```python
from build123d import *

# Parameters (mm, degrees)
SKETCH_1_W      = 119.86
SKETCH_1_H      = 5.07
SKETCH_1_W_2    = 40.6
SKETCH_1_W_3    = 66.26
EXTRUDE_1_DEPTH = 5


with BuildPart() as part:
    # ｽｹｯﾁ1 → ﾎﾞｽ - 押し出し1 (new body)
    with BuildSketch(Plane.XY):
        Polygon((0, 25), (0, 0), (20, 0), (60.6, 0), (60.6, 5.93), (73.6, 5.93), (73.6, 0), (139.86, 0), (164.93, 0), (164.93, 25), (139.86, 25), (20, 25), align=None)
        with Locations((79.93, 27.535)):
            Rectangle(SKETCH_1_W, SKETCH_1_H)
        with Locations((40.3, -2.535)):
            Rectangle(SKETCH_1_W_2, SKETCH_1_H)
        with Locations((106.73, -2.535)):
            Rectangle(SKETCH_1_W_3, SKETCH_1_H)
    extrude(amount=EXTRUDE_1_DEPTH)


solid = part.part
```
Work out the finished part from the listing and answer in its coordinate system (mm). A direction names the side the tool comes from. Give positions to 0.01 mm unless a question says otherwise; leave off trailing zeros. Loops run counter-clockwise (first coordinate to the right, second up) from the corner with the lowest first, then second, coordinate; pieces in that order, holes last. Notation, with made-up numbers: (7, -15) -> (30, -15) arc R24 cw to (30, 13) -> close; hole circle Ø10 at (-5.75, 5). An arc over 180 degrees is marked (long way). Put each result on its own line as item: value. Start each with the question number.
Item 1: Find the intervals of material crossed by L1, parallel to X at y = 3, z = 0.75; L2, parallel to X at y = -3, z = 3.8; L3, parallel to X at y = 25.5, z = 3.75, in increasing order. Write a range as [from, to].
Item 2: The part is cut by section B-B (x = 154). Give the vertices of the cut face in (y, z).
Item 3: Each of these flat-tipped pins is pushed along its axis until it touches: P1, Ø1.5, axis at y = 28, z = 3.5, coming from the +X side; P2, Ø2.5, axis at y = 28.5, z = 2, coming from the -X side. Where does it stop, or does it pass through?
Item 4: Which of the six approach directions +Z, -Z, +X, -X, +Y, -Y give full straight-line access (tool end or side, diameter ignored) to faces 1 (the face through (10, 0, 2)), 2 (the face through (67, 5.93, 2)), 3 (the face through (153, 25, 2))?
Item 5: The mould has two halves that part along X. Classify faces 4 (the face through (60.6, 0, 2)), 5 (the face through (10, 25, 2)), 6 (the face through (139.86, -3, 2)): released by +X, released by -X, zero draft, split by the parting line, or undercut.
Item 6: The part is cut by section C-C (x = 65). Give the vertices of the cut face in (y, z).
Item 7: The part is cut by section A-A (z = 4.25). Give the vertices of the cut face in (x, y), then the cut area to 3 significant figures.
Answers below:
1. L1: [0, 60.6], [73.6, 164.93]
1. L2: [20, 60.6], [73.6, 139.86]
1. L3: [20, 139.86]
2. outline: (0, 0) -> (25, 0) -> (25, 5) -> (0, 5) -> close
3. P1: x = 139.86
3. P2: x = 20
4. face 1: +Z, -Z, -X, -Y
4. face 2: +Z, -Z, -Y
4. face 3: +Z, -Z, +X, +Y
5. face 4: undercut
5. face 5: zero draft
5. face 6: released by +X
6. outline: (5.93, 0) -> (30.07, 0) -> (30.07, 5) -> (5.93, 5) -> close
7. outline: (0, 0) -> (20, 0) -> (20, -5.07) -> (60.6, -5.07) -> (60.6, 5.93) -> (73.6, 5.93) -> (73.6, -5.07) -> (139.86, -5.07) -> (139.86, 0) -> (164.93, 0) -> (164.93, 25) -> (139.86, 25) -> (139.86, 30.07) -> (20, 30.07) -> (20, 25) -> (0, 25) -> close
7. area: 5,200 mm2
